Design review of the part built by this model. Coordinates are the model's own, in mm. A direction names the side the tool comes from. Give positions to 0.01 mm unless a question says otherwise; leave off trailing zeros. Write each loop counter-clockwise with the first axis right and the second up, starting at its lowest first coordinate (ties: lowest second). Pieces come first, ordered by that corner, then holes. Notation, with made-up numbers: M 78.25,34.5 L 123.25,34.5 A12 cw 123.25,48.5 Z; hole C 19,-31.5 d5. An arc over 180 degrees is marked long. Use one line per item in the form item = value. Start each with the question number.
Autodesk Inventor part; units mm, degrees
ref_plane "Начальная плоскость" through (0, 0, 58.9006) normal (0, 0, 1) x (1, 0, 0)
ref_plane "Конечная плоскость" through (0, 0, 458.193) normal (0, 0, 1) x (1, 0, 0)
ref_plane "РабПлоскость8" through (0, 285.6248, -184.0264) normal (0, -0.6924238, -0.721491) x (1, 0, 0)
ref_plane "Начальная плоскость" through (0, 0, 58.9006) normal (0, 0, 1) x (1, 0, 0)
ref_plane "Конечная плоскость" through (0, 0, 458.193) normal (0, 0, 1) x (1, 0, 0)
sketch "Эскиз" plane through (0, 0, 0) normal (0, 0, 1) x (1, 0, 0)
  line L0 (36, -32.5) -> (0, -32.5)
  line L1 (36, -32.5) -> (36, -28.696)
  line L2 (33.6994, -26.2039) -> (9.9215, -24.3017)
  line L3 (4.4, -18.3208) -> (4.4, 18.3208)
  line L4 (33.6994, 26.2039) -> (9.9215, 24.3017)
  line L5 (36, 28.696) -> (36, 32.5)
  line L6 (0, 32.5) -> (36, 32.5)
  line L7 (0, -32.5) -> (0, 32.5)
  arc A0 (4.4, -18.3208) -> (9.9215, -24.3017) centre (10.4, -18.3208) ccw
  arc A1 (9.9215, 24.3017) -> (4.4, 18.3208) centre (10.4, 18.3208) ccw
  arc A2 (36, -28.696) -> (33.6994, -26.2039) centre (33.5, -28.696) ccw
  arc A3 (33.6994, 26.2039) -> (36, 28.696) centre (33.5, 28.696) ccw
  line L8 (0, 45.5) -> (0, -45.5) construction
  line L9 (-7.2974, 0) -> (43.7847, 0) construction
  point P0 (36, -26.388)
  point P1 (4.4, -23.86)
  point P2 (4.4, 23.86)
  point P3 (36, 26.388)
  dimension "d3" = 36
  dimension "d5" = 4.4
  dimension "d7" = 65
  dimension "d9" = 8.64
  dimension "d11" = 8.64
  dimension "d13" = 6.112
  dimension "d15" = 6.112
  dimension "d22" = 6
  dimension "d23" = 2.5
  dimension "d24" = 32.5
  dimension "d25" = 0
extrude "Тело" add sketch "Эскиз" along normal up to surface (399.2924 mm away) from surface at 58.9006
sketch "Sketch3" plane through (0, 0, 0) normal (0, 0, 1) x (1, 0, 0)
  line L0 (0, 0) -> (10, 0)
ref_plane "Work Plane7" through (0, 0, 0) normal (0, -1, 0) x (1, 0, 0)
sketch "Sketch4" plane through (0, 0, 0) normal (0, -1, 0) x (1, 0, 0)
  line L0 (-2, 58.9006) -> (12, 58.9006)
  line L1 (-2, 458.193) -> (12, 458.193)
  dimension "d29" = 399.2924
ref_plane "РабПлоскость8" through (0, 285.6248, -184.0264) normal (0, -0.6924238, -0.721491) x (1, 0, 0)
split "Разделение1" plane through (0, 285.6248, -184.0264) removes the side toward (0, -0.6924238, -0.721491)
ref_plane "РабПлоскость9" through (36, 458.7307, -3.6537) normal (0, 0.6924238, 0.721491) x (1, 0, 0)
split "Разделение2" plane through (36, 458.7307, -3.6537) removes the side toward (0, 0.6924238, 0.721491)
ref_plane "РабПлоскость10" through (-29, 195.6464, 685.5009) normal (0, -0.721491, 0.6924238) x (1, 0, 0)
split "Разделение3" plane through (-29, 195.6464, 685.5009) removes the side toward (0, -0.721491, 0.6924238)
equation "\"d3\" = b"
equation "\"d7\" = ParH"
equation "\"d22\" = R"
equation "\"d23\" = R1"
equation "\"d24\" = 0.5 * d7"
equation "\"d16\" = G_L"
equation "\"R1\" = 2.5"
equation "\"R\" = 6"
equation "\"t1\" = 4.4"
equation "\"t2\" = 7.2"
equation "\"ParH\" = 65"
equation "\"b\" = 36"
equation "\"msp_x1\" = 0.04 * b"
equation "\"msp_x2\" = -0.08 * t1 + 0.04 * b"
equation "\"G_L\" = d29"
equation "\"ex\" = 0"
equation "\"G_OFFSET_START\" = -58.90056"
equation "\"G_OFFSET_END\" = -23.44846"
equation "\"d26\" = -G_OFFSET_START"
equation "\"d27\" = G_OFFSET_END + B_L"
equation "\"B_L\" = 481.64146"
properties part number "Швеллер 6.5U-399,29 ГОСТ 8240-97" material "Сталь, мягкая"
1. For faces 5 (the flat face through (18, -32.5, 282)), 6 (the flat face through (21.977, 25.266, 236.67)), list the 3-axis set-ups (+Z, -Z, +X, -X, +Y, -Y) from which the entire face can be reached by the end or side of a thin tool; tool diameter is ignored.
2. We need section A-A (x = 24). State the section outline as (y, z) points.
3. We need section C-C (y = -8). State the section outline as (x, z) points.
4. Draft analysis for pull direction Y (two halves, no side actions). For faces 1 (the flat face through (21.977, -25.266, 282.466)), 2 (the flat face through (1.9, 0.2, 89.9)), 3 (the flat face through (4.4, 0, 261)), 4 (the flat face through (18, 32.5, 230)), state which applies: pulls with the +Y half, pulls with the -Y half, needs draft (parallel to the pull), parting line crosses it, or undercut.
5. We need section B-B (z = 229.5). State the section outline as (x, y) points.
6. To check wall thickness, follow L1, parallel to Y at x = 9.5, z = 298.5; L2, parallel to X at y = 15, z = 217; L3, parallel to Y at x = 14, z = 401. State the ranges of each line that lie inside material, in increasing order.
7. Clearance check with flat-ended pins moving along their axes: pin 1 Ø11 at (y, z) = (-1, 216) entering from +X; pin 2 Ø3 at (x, y) = (4.5, 23.5) entering from +Z; pin 3 Ø12 at (x, y) = (26.5, 20.5) entering from -Z. State where each tip first meets the part, or that it passes through.
Answer block:
q1.face_5 = +Z, -Z, +X, -X, -Y
q1.face_6 = +Z, -Z, +X
q2.outline = M -32.5,121.28 L -25.43,114.49 L -25.43,455.15 L -32.5,447.78 Z; M 25.43,65.69 L 32.5,58.9 L 32.5,405.41 L 25.43,412.19 Z
q3.outline = M 0,97.77 L 4.4,97.77 L 4.4,444.27 L 0,444.27 Z
q4.face_1 = undercut
q4.face_2 = pulls with the -Y half
q4.face_3 = undercut
q4.face_4 = pulls with the +Y half
q5.outline = M 0,-32.5 L 36,-32.5 L 36,-28.7 A2.5 ccw 33.7,-26.2 L 9.92,-24.3 A6 cw 4.4,-18.32 L 4.4,18.32 A6 cw 9.92,24.3 L 33.7,26.2 A2.5 ccw 36,28.7 L 36,32.5 L 0,32.5 Z
q6.L1 = -32.5 to -24.25, 24.25 to 32.5
q6.L2 = 0 to 4.4
q6.L3 = -32.5 to -24.63, 24.63 to 32.5
q7.pin_1 = 4.4
q7.pin_2 = 415.48
q7.pin_3 = 64.66
